The listing builds one solid part. Answer for the finished solid, in the listing's coordinates (mm). A direction names the side the tool comes from. Round coordinates to 2 decimals unless told otherwise and drop trailing zeros. Order: outer loops, then holes, each group sorted by start corner. A loop starts at its lowest first (then second) coordinate and runs counter-clockwise, first axis right, second up. Notation, with made-up numbers: (1, 48.25) - (45, 48.25) arc R23 cw to (45, 71.25) - close; hole circle Ø1 at (0, -10.75). An arc over 180 degrees is marked (long way). Write item = value, one per line.
from build123d import *

# Parameters (mm, degrees)
SKETCH1_W                    = 32.82
SKETCH1_H                    = 27.07
BOSS_EXTRUDE1_DEPTH          = 12
SKETCH2_W                    = 6
SKETCH2_H                    = 25.07
CUT_EXTRUDE1_DEPTH           = 45.203362994
SKETCH3_W                    = 22.82
SKETCH3_H                    = 12.35
CUT_EXTRUDE2_DEPTH           = 45.203362994
F_2_35_2_35_DIAMETER_HOLE1_D = 2.35
F_2_0_2_DIAMETER_HOLE1_D     = 2


with BuildPart() as part:
    # Sketch1 → Boss-Extrude1 (new body)
    with BuildSketch(Plane(origin=(0, 0, 0), x_dir=(-1, 0, 0), z_dir=(0, 0, -1))):
        with Locations((-16.41, 13.535)):
            Rectangle(SKETCH1_W, SKETCH1_H)
    extrude(amount=-BOSS_EXTRUDE1_DEPTH)

    # Sketch2 → Cut-Extrude1 (cut, through all)
    with BuildSketch(Plane.ZY):
        with Locations((9, 14.535)):
            Rectangle(SKETCH2_W, SKETCH2_H)
    extrude(amount=-CUT_EXTRUDE1_DEPTH, mode=Mode.SUBTRACT)

    # Sketch3 → Cut-Extrude2 (cut, through all)
    with BuildSketch(Plane(origin=(0, 0, 0), x_dir=(-1, 0, 0), z_dir=(0, 0, -1))):
        with Locations((-16.41, 20.895)):
            Rectangle(SKETCH3_W, SKETCH3_H)
    extrude(amount=-CUT_EXTRUDE2_DEPTH, mode=Mode.SUBTRACT)

    # Ø2.35 (2.35) Diameter Hole1 (through all)
    with Locations(Plane.XY.offset(6)):
        with Locations((1.95, 20.87), (30.87, 20.87)):
            Hole(F_2_35_2_35_DIAMETER_HOLE1_D / 2)

    # Ø2.0 (2) Diameter Hole1 (through all)
    with Locations(Plane(origin=(0, 2, 0), x_dir=(1, 0, 0), z_dir=(0, 1, 0))):
        with Locations((28.82, -10), (4, -10)):
            Hole(F_2_0_2_DIAMETER_HOLE1_D / 2)


solid = part.part
Q1. Section D-D on z = 1 is taken. Determine the outline of the cut face in (x, y) (3 decimals).
Model answer:
outline = (0, 0) - (32.82, 0) - (32.82, 27.07) - (27.82, 27.07) - (27.82, 14.72) - (5, 14.72) - (5, 27.07) - (0, 27.07) - close; hole circle Ø2.35 at (1.95, 20.87); hole circle Ø2.35 at (30.87, 20.87)
Q2. Section A-A on z = 10 is taken. Determine the outline of the cut face in (x, y).
Model answer:
outline = (0, 0) - (3, 0) - (3, 2) - (0, 2) - close; (5, 0) - (27.82, 0) - (27.82, 2) - (5, 2) - close; (29.82, 0) - (32.82, 0) - (32.82, 2) - (29.82, 2) - close
Q3. Flat-ended cylindrical pins translate along their axes: P1, Ø3, axis at x = 18.5, y = 3, coming from the +Z side; P2, Ø2, axis at x = 30.87, y = 20.87, coming from the -Z side; P3, Ø1.8, axis at x = 19, z = 7.5, coming from the +Y side; P4, Ø4, axis at x = 1.95, y = 20.87, coming from the +Z side. Find the tip coordinate at first contact, or state that the pin passes through.
Model answer:
P1 = 12
P2 = through
P3 = 2
P4 = 6
Q4. Section B-B on y = 20.87 is taken. Determine the outline of the cut face in (x, z) (3 decimals), then the cut area to 3 significant figures.
Model answer:
outline = (0, 0) - (0.775, 0) - (0.775, 6) - (0, 6) - close; (3.125, 0) - (5, 0) - (5, 6) - (3.125, 6) - close; (27.82, 0) - (29.695, 0) - (29.695, 6) - (27.82, 6) - close; (32.045, 0) - (32.82, 0) - (32.82, 6) - (32.045, 6) - close
area = 31.8 mm^2
Q5. Section C-C on x = 4 is taken. Determine the outline of the cut face in (y, z), then the cut area to 3 significant figures.
Model answer:
outline = (0, 0) - (27.07, 0) - (27.07, 6) - (2, 6) - (2, 9) - (0, 9) - close; (0, 11) - (2, 11) - (2, 12) - (0, 12) - close
area = 170 mm^2
Q6. Find the intervals of material crossed by line 1 (X direction, y = 0.45, z = 10); line 2 (Z direction, x = 4, y = 1.55); line 3 (Z direction, x = 10.5, y = 11.75), in increasing order. Write a range as from..to.
Model answer:
line_1 = 0..3, 5..27.82, 29.82..32.82
line_2 = 0..9, 11..12
line_3 = 0..6
Q7. Determine the mould class of faces 4 (the face through (32.82, 13, 3)), 5 (the face through (28.95, 0.99, 9.01)), 6 (the face through (17, 1, 12)) for opening direction Z: released by +Z, released by -Z, zero draft, split by the parting line, or undercut.
Model answer:
face_4 = zero draft
face_5 = undercut
face_6 = released by +Z
Q8. For faces 1 (the face through (30, 27.07, 3)), 2 (the face through (17, 14.72, 3)), 3 (the face through (16, 2, 9)), determine the directions among +Z, -Z, +X, -X, +Y, -Y from which every point of the face is accessible in a straight line to the end or side of a thin tool.
Model answer:
face_1 = +Z, -Z, +X, -X, +Y
face_2 = +Z, -Z, +Y
face_3 = +Z, +X, -X, +Y
